from build123d import *

# Parameters (mm, degrees)
BOSS_EXTRUDE1_DEPTH       = 8
CUT_EXTRUDE1_DEPTH        = 46
M2X0_4_TAPPED_HOLE1_D     = 1.6
M2X0_4_TAPPED_HOLE1_DEPTH = 5
M2X0_4_TAPPED_HOLE1_TIP   = 0.480688495


with BuildPart() as part:
    # Sketch1 → Boss-Extrude1 (new body)
    with BuildSketch(Plane.XY):
        Polygon((0, 0), (-8, 0), (-8, -20), (-25, -20), (-25, 25), (-8, 25), align=None)
    extrude(amount=BOSS_EXTRUDE1_DEPTH)

    # Sketch2 → Cut-Extrude1 (cut, through all)
    with BuildSketch(Plane(origin=(0, 25, 0), x_dir=(1, 0, 0), z_dir=(0, 1, 0))):
        Polygon((-25, -4), (-25, -1), (-22, -4), (-25, -7), align=None)
    extrude(amount=-CUT_EXTRUDE1_DEPTH, mode=Mode.SUBTRACT)

    # M2x0.4 Tapped Hole1
    with Locations(Plane(origin=(-8, -6, 4), x_dir=(0, 0, 1), z_dir=(1, 0, 0))):
        with Locations((0, 0), (0, 8)):
            Hole(M2X0_4_TAPPED_HOLE1_D / 2, depth=M2X0_4_TAPPED_HOLE1_DEPTH)
            with Locations((0, 0, -(M2X0_4_TAPPED_HOLE1_DEPTH + M2X0_4_TAPPED_HOLE1_TIP / 2))):  # 118° drill point
                Cone(0, M2X0_4_TAPPED_HOLE1_D / 2, M2X0_4_TAPPED_HOLE1_TIP, mode=Mode.SUBTRACT)


solid = part.part
Could you check a few things on this model? Use its own coordinates, in mm. A direction names the side the tool comes from. Coordinates: 2 decimals unless noted, no trailing zeros. Order: outer loops, then holes, each group sorted by start corner. A loop starts at its lowest first (then second) coordinate and runs counter-clockwise, first axis right, second up.
Q1. Please list where these lines run through material, in increasing order: L1, parallel to Y at x = -11.9, z = 4; L2, parallel to Z at x = -11.25, y = -6; L3, parallel to Z at x = -22.75, y = -3.
Q2. Which directions (+Z, -Z, +X, -X, +Y, -Y) give clear straight access to the entire face, cutting with the end or side of a thin tool? Please do faces 4 (the flat face through (-4.056, 12.675, 3.944)), 5 (the flat face through (-24, 3, 2)), 6 (the cylindrical face through (-10.54, -6.54, 4.59)), 7 (the flat face through (-4, 0, 4)).
Q3. Will these pins go through, and if not, where does the flat tip stop? pin 1 (1.4 mm diameter, centred on y = -6, z = 4, fed in from -X); pin 2 (1 mm diameter, centred on y = 14.5, z = 4, fed in from +X); pin 3 (2 mm diameter, centred on y = -14, z = 4, fed in from +X).
Q4. Thinking about a two-plate mould opening in Y: for faces 1 (the flat face through (-16, -20, 4)), 2 (the flat face through (-15, 3, 0)), 3 (the cylindrical face through (-10.535, -14.793, 4.104)), which applies, released by +Y, released by -Y, zero draft, split by the parting line, or undercut?
Q5. Suppose I cut it at C-C on x = -6. Please give me the cut outline in (y, z), and give its area (3 significant figures).
Q6. Suppose I cut it at A-A on x = -22.5. Please give me the cut outline in (y, z).
Q7. Suppose I cut it at D-D on x = -3.25. Please give me the cut outline in (y, z), and give its area (4 significant figures).
Q8. Suppose I cut it at B-B on z = 6.5. Please give me the cut outline in (x, y).
Answer:
1. L1: y = -20 to -14.8, -13.2 to -6.8, -5.2 to 25
1. L2: z = 0 to 3.2, 4.8 to 8
1. L3: z = 0 to 3.25, 4.75 to 8
2. face 4: +Z, -Z, +X, +Y
2. face 5: -X, +Y, -Y
2. face 6: +X
2. face 7: +Z, -Z, +X, -Y
3. pin 1: stops at x = -22.7
3. pin 2: stops at x = -4.48
3. pin 3: stops at x = -8
4. face 1: released by -Y
4. face 2: zero draft
4. face 3: undercut
5. outline: (0, 0) - (18.75, 0) - (18.75, 8) - (0, 8) - close
5. area: 150 mm2
6. outline: (-20, 0) - (25, 0) - (25, 3.5) - (-20, 3.5) - close; (-20, 4.5) - (25, 4.5) - (25, 8) - (-20, 8) - close
7. outline: (0, 0) - (10.16, 0) - (10.16, 8) - (0, 8) - close
7. area: 81.25 mm2
8. outline: (-24.5, -20) - (-8, -20) - (-8, 0) - (0, 0) - (-8, 25) - (-24.5, 25) - close
